Autodesk Inventor part; units mm, degrees
ref_plane "YZ Plane" through (0, 0, 0) normal (1, 0, 0) x (0, 1, 0)
ref_plane "XZ Plane" through (0, 0, 0) normal (0, 1, 0) x (-1, 0, 0)
ref_plane "XY Plane" through (0, 0, 0) normal (0, 0, 1) x (1, 0, 0)
sketch "Sketch14" plane through (0, 0, 0) normal (0, 1, 0) x (-1, 0, 0)
  arc A0 (20, 2.5) -> (20, -2.5) centre (20, 0) ccw
  arc A1 (-2.5, 20) -> (2.5, 20) centre (0, 20) ccw
  arc A2 (-20, -2.5) -> (-20, 2.5) centre (-20, 0) ccw
  arc A3 (2.5, -20) -> (-2.5, -20) centre (0, -20) ccw
  line L0 (20, -2.5) -> (15.8035, -2.5)
  line L1 (20, 2.5) -> (15.8035, 2.5)
  line L2 (2.5, 20) -> (2.5, 15.8035)
  line L3 (-2.5, 20) -> (-2.5, 15.8035)
  line L4 (-20, 2.5) -> (-15.8035, 2.5)
  line L5 (-20, -2.5) -> (-15.8035, -2.5)
  line L6 (-2.5, -20) -> (-2.5, -15.8035)
  line L7 (2.5, -20) -> (2.5, -15.8035)
  arc A4 (2.5, -15.8035) -> (15.8035, -2.5) centre (0, 0) ccw
  arc A5 (15.8035, 2.5) -> (2.5, 15.8035) centre (0, 0) ccw
  arc A6 (-2.5, 15.8035) -> (-15.8035, 2.5) centre (0, 0) ccw
  arc A7 (-15.8035, -2.5) -> (-2.5, -15.8035) centre (0, 0) ccw
  circle A8 centre (0, 0) radius 7.5
  dimension "d87" = 2.5
  dimension "d88" = 2.5
  dimension "d89" = 2.5
  dimension "d90" = 2.5
  dimension "d91" = 15
extrude "Extrusion15" add sketch "Sketch14" along normal blind 5
sketch "Sketch15" plane through (0, 0, 0) normal (0, -1, 0) x (1, 0, 0)
  circle A0 centre (0, 0) radius 8.5
  circle A1 centre (0, 0) radius 15
  dimension "d94" = 17
  dimension "d95" = 30
extrude "Extrusion16" cut sketch "Sketch15" against normal blind 1
sketch "Sketch16" plane through (0, 5, 0) normal (0, 1, 0) x (1, 0, 0)
  arc A0 (-20, -2.5) -> (-20, 2.5) centre (-20, 0) ccw
  arc A1 (-20, -2.5) -> (-20, 2.5) centre (-20, 0) ccw
  arc A2 (2.5, -20) -> (-2.5, -20) centre (0, -20) ccw
  arc A3 (2.5, -20) -> (-2.5, -20) centre (0, -20) ccw
  arc A4 (20, 2.5) -> (20, -2.5) centre (20, 0) ccw
  arc A5 (-2.5, 20) -> (2.5, 20) centre (0, 20) ccw
  line L0 (-20, 2.5) -> (-14, 2.5)
  line L1 (-14, 2.5) -> (-14, -2.5)
  line L2 (-14, -2.5) -> (-20, -2.5)
  line L3 (-2.5, -15.8035) -> (-2.5, -20)
  line L4 (-2.5, -20) -> (-2.5, -14)
  line L5 (-2.5, -14) -> (2.5, -14)
  line L6 (2.5, -20) -> (2.5, -15.8035)
  line L7 (2.5, -14) -> (2.5, -20)
  line L8 (20, -2.5) -> (14, -2.5)
  line L9 (15.8035, -2.5) -> (20, -2.5)
  line L10 (14, -2.5) -> (14, 2.5)
  line L11 (20, 2.5) -> (15.8035, 2.5)
  line L12 (14, 2.5) -> (20, 2.5)
  line L13 (2.5, 15.8035) -> (2.5, 20)
  line L14 (2.5, 20) -> (2.5, 14)
  line L15 (2.5, 14) -> (-2.5, 14)
  arc A6 (-2.5, 20) -> (2.5, 20) centre (0, 20) ccw
  line L16 (-2.5, 14) -> (-2.5, 20)
  point P0 (0, 0)
extrude "Extrusion17" add sketch "Sketch16" along normal blind 8
sketch "Sketch17" plane through (0, 13, 0) normal (0, 1, 0) x (1, 0, 0)
  line L0 (-2.5, 20) -> (-2.5, 15.8035)
  arc A0 (-2.5, 20) -> (2.5, 20) centre (0, 20) ccw
  arc A1 (-2.5, 20) -> (2.5, 20) centre (0, 20) ccw
  arc A2 (20, 2.5) -> (20, -2.5) centre (20, 0) ccw
  arc A3 (20, 2.5) -> (20, -2.5) centre (20, 0) ccw
  arc A4 (2.5, -20) -> (-2.5, -20) centre (0, -20) ccw
  line L1 (-20, -2.5) -> (-2.5, -2.5)
  line L2 (-2.5, -2.5) -> (-2.5, -20)
  line L3 (2.5, -20) -> (2.5, -2.5)
  line L4 (2.5, -2.5) -> (20, -2.5)
  line L5 (20, 2.5) -> (2.5, 2.5)
  line L6 (2.5, 15.8035) -> (2.5, 20)
  line L7 (2.5, 2.5) -> (2.5, 20)
  line L8 (-2.5, 20) -> (-2.5, 2.5)
  line L9 (-20, 2.5) -> (-2.5, 2.5)
  arc A5 (-20, -2.5) -> (-20, 2.5) centre (-20, 0) ccw
  point P0 (0, 0)
extrude "Extrusion18" add sketch "Sketch17" along normal blind 4
sketch "Sketch18" plane through (0, 17, 0) normal (0, 1, 0) x (1, 0, 0)
  circle A0 centre (0, 0) radius 1
  dimension "d102" = 2
extrude "Extrusion19" add sketch "Sketch18" along normal blind 4
fillet "Fillet1" radius 2 5 edges at (11.3137, 5, -11.3137) (7.5, 5, 0) (-11.3137, 5, -11.3137) (-11.3137, 5, 11.3137) (11.3137, 5, 11.3137)
fillet "Fillet2" radius 2 1 edges at (-1, 17, 0)
properties part number "CheckValveValve1.0"
CAD build for the part. Positions are in the model's coordinates, mm. A direction names the side the tool comes from. Coordinates: 2 decimals unless noted, no trailing zeros. Write each loop counter-clockwise with the first axis right and the second up, starting at its lowest first coordinate (ties: lowest second). Pieces come first, ordered by that corner, then holes.
(1) Two-plate mould, pull along Z, no slides. Class faces 6 (the face through (-15, 10, -2.5)), 7 (the face through (0, 9, 14)), 8 (the face through (0, 20, -1)), 9 (the face through (2.5, 10, -15)): +Z half, -Z half, draft (parallel to the pull), parting line (faces both ways), or undercut.
(2) Cut at A-A, the plane y = 8. List the corners of the cut face in (x, z), and give its area (3 significant figures).
(3) Cut at B-B, the plane z = 3.5. Count the separate pieces of the cut face and the enclosed holes in it, and give its area (3 significant figures).
(4) Drill centre lines: probe 1 along Z at (x, y) = (0, 0.6); probe 2 along Y at (x, z) = (0, 9.5); probe 3 along X at (y, z) = (4, -17). Where is each one in solid material? Low to high.
(5) 3-axis set-ups, long thin cutter, end or side, ignore diameter. For faces 1 (the face through (-14.985, 0.493, 0.66)), 2 (the face through (15, 10, 2.5)), 3 (the face through (-1, 13, 0)), 4 (the face through (15, 10, -2.5)), 5 (the face through (14, 9, 0)): which of +Z, -Z, +X, -X, +Y, -Y reach the whole face in a straight line?
(6) Flat gauge pins, fed straight in: pin 1 (1 mm diameter, centred on x = 5.5, z = 4.5, fed in from -Y); pin 2 (3 mm diameter, centred on x = 6, z = 4.5, fed in from +Y); pin 3 (8 mm diameter, centred on x = 5.5, z = -6, fed in from +Y); pin 4 (8.5 mm diameter, centred on x = 14.5, y = 8, fed in from +Z). Where does each tip first touch, or does it go through?
Geometry says:
1. face 6: -Z half
1. face 7: undercut
1. face 8: parting line
1. face 9: draft
2. outline: (-20, -2.5) - (-14, -2.5) - (-14, 2.5) - (-20, 2.5) arc R2.5 cw to start; (-2.5, -20) arc R2.5 cw to (2.5, -20) - (2.5, -14) - (-2.5, -14) - close; (-2.5, 14) - (2.5, 14) - (2.5, 20) arc R2.5 cw to (-2.5, 20) - close; (14, -2.5) - (20, -2.5) arc R2.5 cw to (20, 2.5) - (14, 2.5) - close
2. area: 80.7 mm2
3. separate pieces: 3
3. enclosed holes: 0
3. area: 92.4 mm2
4. probe 1: z = -17.5 to -15, -8.5 to -7.5, 7.5 to 8.5, 15 to 17.5
4. probe 2: y = 1 to 5, 13 to 17
4. probe 3: x = -2.5 to 2.5
5. face 1: -Y
5. face 2: +Z, +X, +Y
5. face 3: none
5. face 4: -Z, +X, +Y
5. face 5: +Z, -Z
6. pin 1: stops at y = 0
6. pin 2: stops at y = 4.94
6. pin 3: stops at y = 17
6. pin 4: stops at z = 9.42
